Part model, mm, in its own coordinate system. Face numbers are marked on the shaded views. A direction names the side the tool comes from. Round coordinates to 2 decimals unless told otherwise and drop trailing zeros. Loops run counter-clockwise (first coordinate to the right, second up) from the corner with the lowest first, then second, coordinate; pieces in that order, holes last. Notation, with made-up numbers: (67.5, 83.25) -> (105.5, 83.25) arc R11 ccw to (105.5, 100.25) -> close; hole circle Ø10 at (-2.75, 57). An arc over 180 degrees is marked (long way). Answer as a JSON object with one key per item and string values. Group by question number.
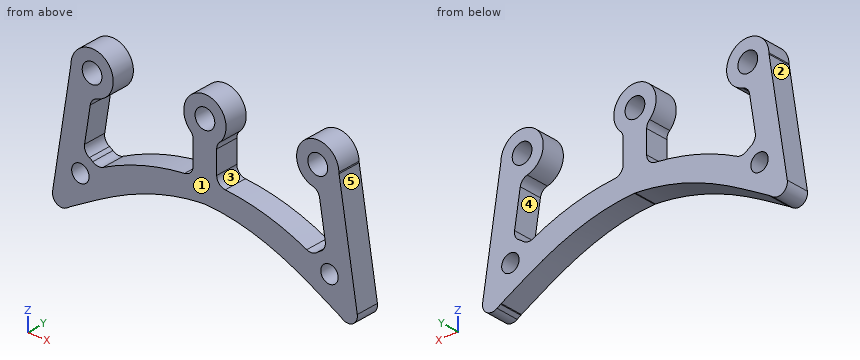
from build123d import *

# Parameters (mm, degrees)
SKETCH1_R           = 2.1
SKETCH1_R_2         = 1.85
BOSS_EXTRUDE1_DEPTH = 5
FILLET1_R           = 2


with BuildPart() as part:
    # Sketch1 → Boss-Extrude1 (new body)
    with BuildSketch(Plane(origin=(0, 0, 0), x_dir=(1, 0, 0), z_dir=(0, 1, 0))):
        with BuildLine():
            Line((64.703578791, 22.153935156), (60.086593503, -6.943643112))
            ThreePointArc((60.086593503, -6.943643112), (52.351867725, -10.071989183), (55.737016108, -2.446157921))
            Line((55.737016108, -2.446157921), (57.44284906, 8.304495315))
            ThreePointArc((57.44284906, 8.304495315), (55.811241442, 8.948588976), (54.605866, 10.222979068))
            ThreePointArc((54.605866, 10.222979068), (44.668654946, 6.187635781), (34.085703384, 4.445999995))
            Line((34.085703384, 4.445999995), (34.085703384, -3.201391143))
            ThreePointArc((34.085703384, -3.201391143), (31.586593503, -11.443643112), (29.087483622, -3.201391143))
            Line((29.087483622, -3.201391143), (29.087483622, 4.445999995))
            ThreePointArc((29.087483622, 4.445999995), (18.504532059, 6.187635781), (8.567321006, 10.222979068))
            ThreePointArc((8.567321006, 10.222979068), (7.361945564, 8.948588976), (5.730337946, 8.304495315))
            Line((5.730337946, 8.304495315), (7.436170898, -2.446157921))
            ThreePointArc((7.436170898, -2.446157921), (10.821319281, -10.071989183), (3.086593503, -6.943643112))
            Line((3.086593503, -6.943643112), (-1.530391785, 22.153935156))
            Line((-1.530391785, 22.153935156), (3.086593503, 19.066758984))
            add(Edge.make_bspline(
                [(3.086593503, 19.066758984), (6.214599524, 17.320565922), (15.289655428, 11.953978367), (24.991497583, 9.011909138), (31.586593503, 8.723848672)],
                knots=[0.224841934, 0.224841934, 0.224841934, 0.224841934, 0.497996304, 1, 1, 1, 1], degree=3))
            add(Edge.make_bspline(
                [(60.086593503, 19.066758984), (56.958587482, 17.320565922), (47.883531578, 11.953978367), (38.181689422, 9.011909138), (31.586593503, 8.723848672)],
                knots=[0.224841934, 0.224841934, 0.224841934, 0.224841934, 0.497996304, 1, 1, 1, 1], degree=3))
            Line((60.086593503, 19.066758984), (64.703578791, 22.153935156))
        make_face()
        with Locations(Location((7.586593503, -6.943643112, 0), (0, 0, 270))):
            Circle(SKETCH1_R, mode=Mode.SUBTRACT)
        with Locations(Location((55.586593503, -6.943643112, 0), (0, 0, 90))):
            Circle(SKETCH1_R, mode=Mode.SUBTRACT)
        with Locations(Location((31.586593503, -6.943643112, 0), (0, 0, 270))):
            Circle(SKETCH1_R, mode=Mode.SUBTRACT)
        with Locations(Location((5.096599352, 12.298499455, 0), (0, 0, 270))):
            Circle(SKETCH1_R_2, mode=Mode.SUBTRACT)
        with Locations(Location((58.076587654, 12.298499455, 0), (0, 0, 270))):
            Circle(SKETCH1_R_2, mode=Mode.SUBTRACT)
    extrude(amount=BOSS_EXTRUDE1_DEPTH)

    # Fillet1
    # the kernel refuses this fillet: 2 mm, written as the material it adds along each edge
    with BuildSketch(Plane(origin=(60.086593503, 0, 6.943643112), x_dir=(0.15671199054579144, 0, -0.9876443449031517), z_dir=(0, 1, 0))) as fillet1_piece_1:
        with BuildLine():
            CenterArc((0.14315588, -2), FILLET1_R, 90, 7.499462887)
            ThreePointArc((-0.117877916, -0.01710783), (-0.058882351, -0.008943954), (0, 0))
            Line((0, 0), (0.14315588, 0))
        make_face()
    extrude(amount=5)
    with BuildSketch(Plane(origin=(55.737016108, 0, 2.446157921), x_dir=(-0.9943134943930577, 0, 0.1064926047566996), z_dir=(0, 1, 0))) as fillet1_piece_2:
        with BuildLine():
            CenterArc((1.536372783, -1.980396143), FILLET1_R, 98.028765666, 66.841966003)
            Line((-0.39430608, -1.458400811), (0, 0))
            ThreePointArc((0, 0), (0.628516139, -0.044108679), (1.257032277, 0))
        make_face()
    extrude(amount=5)
    with BuildSketch(Plane(origin=(57.44284906, 0, -8.304495315), x_dir=(-0.15671199054619364, 0, 0.9876443449030878), z_dir=(0, 1, 0))) as fillet1_piece_3:
        with BuildLine():
            CenterArc((1.659500293, -2), FILLET1_R, 90, 70.676083633)
            ThreePointArc((-0.227825519, -1.338183351), (-0.057363225, -0.678719225), (0, 0))
            Line((0, 0), (1.659500293, 0))
        make_face()
    extrude(amount=5)
    with BuildSketch(Plane(origin=(54.605866, 0, -10.222979068), x_dir=(0.6436684340700369, 0, 0.7653044799175203), z_dir=(0, 1, 0))) as fillet1_piece_4:
        with BuildLine():
            CenterArc((1.610462564, -1.974349834), FILLET1_R, 99.186138147, 67.391276413)
            ThreePointArc((-0.334906336, -1.510087145), (-0.161404643, -0.756385011), (0, 0))
            ThreePointArc((0, 0), (0.645588922, -0.051864251), (1.291177843, 0))
        make_face()
    extrude(amount=5)
    with BuildSketch(Plane(origin=(34.085703384, 0, -4.445999995), x_dir=(0, 0, 1), z_dir=(0, 1, 0))) as fillet1_piece_5:
        with BuildLine():
            CenterArc((1.863012192, 2), FILLET1_R, 185.134308641, 84.865691359)
            ThreePointArc((-0.128963122, 1.821018582), (-0.055872709, 0.911118963), (0, 0))
            Line((0, 0), (1.863012192, 0))
        make_face()
    extrude(amount=5)
    with BuildSketch(Plane(origin=(34.085703384, 0, 3.201391143), x_dir=(0, 0, -1), z_dir=(0, 1, 0))) as fillet1_piece_6:
        with BuildLine():
            CenterArc((0.949017611, -2), FILLET1_R, 90, 46.197810795)
            ThreePointArc((-0.494449952, -0.615658498), (-0.233694925, -0.318695554), (0, 0))
            Line((0, 0), (0.949017611, 0))
        make_face()
    extrude(amount=5)
    with BuildSketch(Plane(origin=(29.087483622, 0, 3.201391143), x_dir=(-0.7796793430593535, 0, 0.6261789855995925), z_dir=(0, 1, 0))) as fillet1_piece_7:
        with BuildLine():
            CenterArc((0.965103801, -1.992287399), FILLET1_R, 95.03341493, 46.197810795)
            Line((-0.594254885, -0.739929428), (0, 0))
            ThreePointArc((0, 0), (0.394815191, -0.017353353), (0.789630383, 0))
        make_face()
    extrude(amount=5)
    with BuildSketch(Plane(origin=(29.087483622, 0, -4.445999995), x_dir=(0, 0, 1), z_dir=(0, 1, 0))) as fillet1_piece_8:
        with BuildLine():
            CenterArc((1.863012192, -2), FILLET1_R, 90, 84.865691359)
            ThreePointArc((-0.128963122, -1.821018582), (-0.055872709, -0.911118963), (0, 0))
            Line((0, 0), (1.863012192, 0))
        make_face()
    extrude(amount=5)
    with BuildSketch(Plane(origin=(5.730337946, 0, -8.304495315), x_dir=(0.9473329914518264, 0, -0.3202502198390094), z_dir=(0, 1, 0))) as fillet1_piece_9:
        with BuildLine():
            CenterArc((1.69310821, -1.971630242), FILLET1_R, 99.661958184, 70.676083633)
            Line((-0.278522032, -1.635960483), (0, 0))
            ThreePointArc((0, 0), (0.678719225, -0.057363225), (1.357438451, 0))
        make_face()
    extrude(amount=5)
    with BuildSketch(Plane(origin=(7.436170898, 0, 2.446157921), x_dir=(-0.15671199054620055, 0, -0.987644344903087), z_dir=(0, 1, 0))) as fillet1_piece_10:
        with BuildLine():
            CenterArc((1.510764777, -2), FILLET1_R, 90, 66.841966003)
            ThreePointArc((-0.32808249, -1.213462824), (-0.121461398, -0.618243674), (0, 0))
            Line((0, 0), (1.510764777, 0))
        make_face()
    extrude(amount=5)
    with BuildSketch(Plane(origin=(3.086593503, 0, 6.943643112), x_dir=(0.013234765762904084, 0, 0.9999124166521791), z_dir=(0, 1, 0))) as fillet1_piece_11:
        with BuildLine():
            CenterArc((0.145582423, -1.999824833), FILLET1_R, 90.75831836, 7.499462887)
            Line((-0.141671624, -0.020561053), (0, 0))
            ThreePointArc((0, 0), (0.059556446, -0.000394125), (0.119112892, 0))
        make_face()
    extrude(amount=5)
    with BuildSketch(Plane(origin=(3.086593503, 0, -19.066758984), x_dir=(-0.831286153352586, 0, -0.5558447006532138), z_dir=(0, 1, 0))) as fillet1_piece_12:
        with BuildLine():
            CenterArc((0.080080644, -2), FILLET1_R, 90, 4.575133674)
            ThreePointArc((-0.079451987, -0.006372818), (-0.039725694, -0.003190148), (0, 0))
            Line((0, 0), (0.080080644, 0))
        make_face()
    extrude(amount=5)
    with BuildSketch(Plane(origin=(31.586593503, 0, -8.723848672), x_dir=(-0.9989968341104656, 0, -0.044780860166667026), z_dir=(0, 1, 0))) as fillet1_piece_13:
        with BuildLine():
            CenterArc((0.089651597, -1.999998688), FILLET1_R, 89.934377151, 5.264470885)
            ThreePointArc((-0.091573518, -0.008226247), (-0.045789115, -0.0040869), (0, 0))
            ThreePointArc((0, 0), (0.045971133, 2.6329e-05), (0.091942266, 0))
        make_face()
    extrude(amount=5)
    with BuildSketch(Plane(origin=(60.086593503, 0, -19.066758984), x_dir=(-0.8730663040204696, 0, 0.4876015061338889), z_dir=(0, 1, 0))) as fillet1_piece_14:
        with BuildLine():
            CenterArc((0.080081519, -1.999999965), FILLET1_R, 90.010724643, 4.575133674)
            Line((-0.079824277, -0.00640268), (0, 0))
            ThreePointArc((0, 0), (0.039853579, -3.751e-06), (0.079707158, 0))
        make_face()
    extrude(amount=5)
    with BuildSketch(Plane(origin=(8.567321006, 0, -10.222979068), x_dir=(0.8865164621041475, 0, 0.46269705252826665), z_dir=(0, 1, 0))) as fillet1_piece_15:
        with BuildLine():
            CenterArc((1.578820312, -1.999743323), FILLET1_R, 90.91795372, 67.391276413)
            ThreePointArc((-0.279563936, -1.260549177), (-0.089148014, -0.64150416), (0, 0))
            ThreePointArc((0, 0), (0.773389527, -0.006195491), (1.546779054, 0))
        make_face()
    extrude(amount=5)
    # the kernel refuses this fillet: 2 mm, written as the material it takes off along each edge
    with BuildSketch(Plane(origin=(64.703578791, -11.440469637, -22.153935156), x_dir=(-0.831286153352585, 0, 0.5558447006532152), z_dir=(0, 1, 0)), Plane(origin=(-1.530391785, -11.440469637, -22.153935156), x_dir=(0.15671199054620674, 0, 0.987644344903086), z_dir=(0, 1, 0))) as fillet1_2_piece_1:
        with BuildLine():
            CenterArc((FILLET1_R * 2.28809392748, FILLET1_R), FILLET1_R, 137.214985003, 132.785014997)
            Line((FILLET1_R * 1.5541863886, FILLET1_R * 1.67924938305), (0, 0))
            Line((0, 0), (FILLET1_R * 2.28809392748, 0))
        make_face()
    extrude(amount=27.880939275, mode=Mode.SUBTRACT)


solid = part.part
Item 1: Drop flat-ended pins along their axis: pin 1 Ø4 at (x, z) = (7.59, 6.94) entering from -Y; pin 2 Ø1.5 at (y, z) = (2.5, -1) entering from -X; pin 3 Ø3 at (y, z) = (1, -2) entering from -X; pin 4 Ø1 at (x, y) = (6, 0.5) entering from +Z. Give the stop position or say it passes through.
Item 2: Which spindle directions (+Z, -Z, +X, -X, +Y, -Y) get a long thin tool onto all of the face, cutting with end or side? Do the marked faces 4 and 5. Say none if no direction does.
Item 3: Two-plate mould, pull along Z, no slides. Class the marked faces 1, 2 and 3: pulls with the +Z half, pulls with the -Z half, needs draft (parallel to the pull), parting line crosses it, or undercut.
Item 4: Band-saw the part on B-B, the plane y = 1.1. Count the separate pieces of the cut face and the enclosed holes in it, plus the area to 3 significant figures.
Item 5: Band-saw the part on A-A, the plane z = -1. List the corners of the cut face in (x, y), plus the area to 3 significant figures.
Item 6: Drill centre lines: line 1 (X direction, y = 3.65, z = 3); line 2 (X direction, y = 2.05, z = -3); line 3 (X direction, y = 1.1, z = 7.5). Where is each one in solid material? Low to high.
Entries:
{
 "1": {"pin 1": "through", "pin 2": "x = 1.71", "pin 3": "x = 1.43", "pin 4": "z = 11.31"},
 "2": {"face 4": "+Y, -Y", "face 5": "+Z, +X, +Y, -Y"},
 "3": {"face 1": "needs draft", "face 2": "pulls with the +Z half", "face 3": "undercut"},
 "4": {"separate pieces": "1", "enclosed holes": "5", "area": "693 mm²"},
 "5": {"outline": "(1.83, 0) -> (6.89, 0) -> (6.89, 5) -> (1.83, 5) -> close; (29.09, 0) -> (34.09, 0) -> (34.09, 5) -> (29.09, 5) -> close; (56.28, 0) -> (61.35, 0) -> (61.35, 5) -> (56.28, 5) -> close", "area": "75.6 mm²"},
 "6": {"line 1": "2.46 to 9.75, 28.94 to 34.23, 53.42 to 60.71", "line 2": "1.51 to 6.57, 29.04 to 34.13, 56.6 to 61.66", "line 3": "3.12 to 5.56, 9.61 to 12.05, 27.12 to 29.56, 33.61 to 36.05, 51.12 to 53.56, 57.61 to 60.05"}
}
